The listing builds one solid part. Answer for the finished solid, in the listing's coordinates (mm). Face numbers are marked on the shaded views. A direction names the side the tool comes from. Give positions to 0.01 mm unless a question says otherwise; leave off trailing zeros. Write each loop counter-clockwise with the first axis right and the second up, starting at its lowest first coordinate (ties: lowest second). Pieces come first, ordered by that corner, then holes. Notation, with made-up numbers: M -14,28 L -8,28 A29 ccw -8,61 Z; hole C 1.5,-36.5 d11. An arc over 180 degrees is marked long. Answer as a JSON object with one key per item and string values.
```python
from build123d import *

# Parameters (mm, degrees)
EXTRUDE_1_DEPTH     = 10
CUT_EXTRUDE_1_DEPTH = 6
FILLET_1_R          = 2
SKETCH_3_R          = 5
CUT_EXTRUDE_2_DEPTH = 6
SKETCH_5_R          = 4
CUT_EXTRUDE_3_DEPTH = 94.307288033


with BuildPart() as part:
    # 草图1 → 凸台-拉伸1 (new body)
    with BuildSketch(Plane.XY):
        with BuildLine():
            Line((-22.5, 0), (-22.5, -87))
            ThreePointArc((-22.5, -87), (-21.621320344, -89.121320344), (-19.5, -90))
            Line((-19.5, -90), (19.5, -90))
            ThreePointArc((19.5, -90), (21.621320344, -89.121320344), (22.5, -87))
            Line((22.5, -87), (22.5, 0))
            ThreePointArc((22.5, 0), (0, 22.5), (-22.5, 0))
        make_face()
    extrude(amount=EXTRUDE_1_DEPTH)

    # 草图2 → 切除-拉伸1 (cut)
    with BuildSketch(Plane(origin=(0, 0, 0), x_dir=(-1, 0, 0), z_dir=(0, 0, -1))):
        with BuildLine():
            Line((-22.5, 0), (-22.5, -27.5))
            Line((-22.5, -27.5), (22.5, -27.5))
            Line((22.5, -27.5), (22.5, 0))
            ThreePointArc((22.5, 0), (15.909902614, 15.909902539), (1.06e-07, 22.5))
            ThreePointArc((1.06e-07, 22.5), (-15.909902539, 15.909902614), (-22.5, 0))
        make_face()
    extrude(amount=-CUT_EXTRUDE_1_DEPTH, mode=Mode.SUBTRACT)

    # 圆角1
    fillet_1_edges = [part.edges().sort_by_distance(p)[0] for p in [
        (0, -27.5, 0),
    ]]
    fillet(fillet_1_edges, radius=FILLET_1_R)

    # 草图3 → 切除-拉伸2 (cut)
    with BuildSketch(Plane.XY.offset(10)):
        Circle(SKETCH_3_R)
    extrude(amount=-CUT_EXTRUDE_2_DEPTH, mode=Mode.SUBTRACT)

    # 草图5 → 切除-拉伸3 (cut, through all)
    with BuildSketch(Plane(origin=(0, 0, 0), x_dir=(-1, 0, 0), z_dir=(0, 0, -1))):
        with Locations((-12.5, -44.5)):
            Circle(SKETCH_5_R)
        with Locations((12.5, -44.5)):
            Circle(SKETCH_5_R)
        with Locations((12.5, -75)):
            Circle(SKETCH_5_R)
        with Locations((-12.5, -75)):
            Circle(SKETCH_5_R)
    extrude(amount=-CUT_EXTRUDE_3_DEPTH, mode=Mode.SUBTRACT)


solid = part.part
```
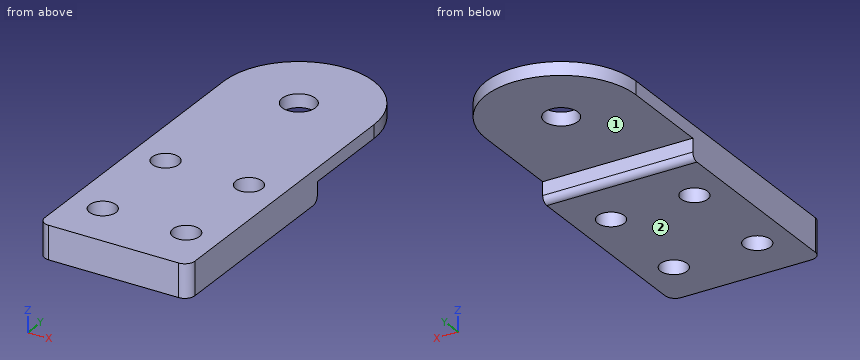
1. For the marked faces 1 and 2, determine the directions among +Z, -Z, +X, -X, +Y, -Y from which every point of the face is accessible in a straight line to the end or side of a thin tool.
Verdict:
{"face 1": "-Z, +X, -X, +Y", "face 2": "-Z, +X, -X, +Y, -Y"}
2. A cutting plane is placed at B-B, the plane z = 8.25. Give the vertices of the cut face in (x, y).
Verdict:
{"outline": "M -22.5,-87 A3 ccw -19.5,-90 L 19.5,-90 A3 ccw 22.5,-87 L 22.5,0 A22.5 ccw -22.5,0 Z; hole C -12.5,-75 d8; hole C -12.5,-44.5 d8; hole C 0,0 d10; hole C 12.5,-75 d8; hole C 12.5,-44.5 d8"}
3. A cutting plane is placed at D-D, the plane x = -3. Give the vertices of the cut face in (y, z).
Verdict:
{"outline": "M -90,0 L -29.5,0 A2 ccw -27.5,2 L -27.5,6 L -4,6 L -4,10 L -90,10 Z; M 4,6 L 22.3,6 L 22.3,10 L 4,10 Z"}
4. A cutting plane is placed at C-C, the plane x = 14. Give the vertices of the cut face in (y, z).
Verdict:
{"outline": "M -90,0 L -78.71,0 L -78.71,10 L -90,10 Z; M -71.29,0 L -48.21,0 L -48.21,10 L -71.29,10 Z; M -40.79,0 L -29.5,0 A2 ccw -27.5,2 L -27.5,6 L 17.61,6 L 17.61,10 L -40.79,10 Z"}
5. A cutting plane is placed at A-A, the plane y = -75. Give the vertices of the cut face in (x, z), plus the area to 3 significant figures.
Verdict:
{"outline": "M -22.5,0 L -16.5,0 L -16.5,10 L -22.5,10 Z; M -8.5,0 L 8.5,0 L 8.5,10 L -8.5,10 Z; M 16.5,0 L 22.5,0 L 22.5,10 L 16.5,10 Z", "area": "290 mm2"}
6. Consider line 1 along Y through (x, z) = (12.5, 3.25); line 2 along Y through (x, z) = (-12.5, 7.5); line 3 along Y through (x, z) = (0, 7.4). Determine where each line is inside the solid, lowest interval first.
Verdict:
{"line 1": "y = -90 to -79, -71 to -48.5, -40.5 to -27.5", "line 2": "y = -90 to -79, -71 to -48.5, -40.5 to 18.71", "line 3": "y = -90 to -5, 5 to 22.5"}
7. Flat-ended cylindrical pins translate along their axes: pin 1 (6 mm diameter, centred on x = -6.5, y = -65, fed in from -Z); pin 2 (1.2 mm diameter, centred on x = -6, z = 4.5, fed in from +Y); pin 3 (13 mm diameter, centred on x = 0, y = 0, fed in from -Z); pin 4 (2 mm diameter, centred on x = 8.5, z = 6, fed in from +Y). Find the tip coordinate at first contact, or state that the pin passes through.
Verdict:
{"pin 1": "stops at z = 0", "pin 2": "stops at y = -27.5", "pin 3": "stops at z = 6", "pin 4": "stops at y = 21.21"}
